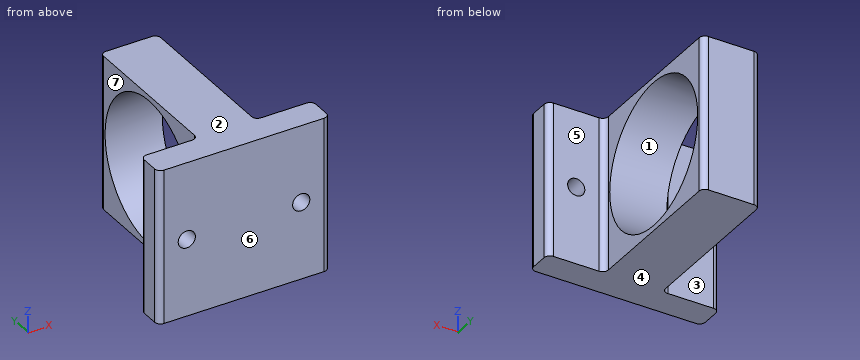
from build123d import *

# Parameters (mm, degrees)
BOSS_EXTRUDE1_DEPTH = 27
CUT_EXTRUDE1_REACH  = 45.738
SKETCH2_R           = 12.6
CUT_EXTRUDE2_REACH  = 47.2
SKETCH3_R           = 1.5


with BuildPart() as part:
    # Sketch1 → Boss-Extrude1 (new body)
    with BuildSketch(Plane.XY):
        with BuildLine():
            Line((-14, 0), (-6, 0))
            ThreePointArc((-6, 0), (-5.292893219, 0.292893219), (-5, 1))
            Line((-5, 1), (-5, 27))
            ThreePointArc((-5, 27), (-4.707106781, 27.707106781), (-4, 28))
            Line((-4, 28), (4, 28))
            ThreePointArc((4, 28), (4.707106781, 27.707106781), (5, 27))
            Line((5, 27), (5, 1))
            ThreePointArc((5, 1), (5.292893219, 0.292893219), (6, 0))
            Line((6, 0), (14, 0))
            ThreePointArc((14, 0), (14.707106781, -0.292893219), (15, -1))
            Line((15, -1), (15, -4))
            ThreePointArc((15, -4), (14.707106781, -4.707106781), (14, -5))
            Line((14, -5), (-14, -5))
            ThreePointArc((-14, -5), (-14.707106781, -4.707106781), (-15, -4))
            Line((-15, -4), (-15, -1))
            ThreePointArc((-15, -1), (-14.707106781, -0.292893219), (-14, 0))
        make_face()
    extrude(amount=BOSS_EXTRUDE1_DEPTH)

    # Sketch2 → Cut-Extrude1 (cut, up to next)
    with BuildSketch(Plane(origin=(5, 0, 0), x_dir=(0, 0, -1), z_dir=(1, 0, 0)), mode=Mode.PRIVATE) as cut_extrude1_sk1:
        with Locations(Location((-13.5, 14, 0), (0, 0, 90))):
            Circle(SKETCH2_R)
    cut_extrude1_tool1 = extrude(cut_extrude1_sk1.sketch, amount=-CUT_EXTRUDE1_REACH, mode=Mode.PRIVATE) & part.part
    add(cut_extrude1_tool1.solids().sort_by_distance((5, 14, 13.5))[0], mode=Mode.SUBTRACT)

    # Sketch3 → Cut-Extrude2 (cut, up to next)
    with BuildSketch(Plane.XZ.offset(5), mode=Mode.PRIVATE) as cut_extrude2_sk1:
        with Locations((-10, 13.5)):
            Circle(SKETCH3_R)
    cut_extrude2_tool1 = extrude(cut_extrude2_sk1.sketch, amount=-CUT_EXTRUDE2_REACH, mode=Mode.PRIVATE) & part.part
    # Sketch3 → Cut-Extrude2 (cut, up to next)
    with BuildSketch(Plane.XZ.offset(5), mode=Mode.PRIVATE) as cut_extrude2_sk2:
        with Locations(Location((10, 13.5, 0), (0, 0, 270))):
            Circle(SKETCH3_R)
    cut_extrude2_tool2 = extrude(cut_extrude2_sk2.sketch, amount=-CUT_EXTRUDE2_REACH, mode=Mode.PRIVATE) & part.part
    add(cut_extrude2_tool1.solids().sort_by_distance((-10, -5, 13.5))[0], mode=Mode.SUBTRACT)
    add(cut_extrude2_tool2.solids().sort_by_distance((10, -5, 13.5))[0], mode=Mode.SUBTRACT)


solid = part.part
Geometry check sheet. Reference: the model listing, model coordinates, mm. Face numbers are marked on the shaded views. A direction names the side the tool comes from. Coordinates: 2 decimals unless noted, no trailing zeros. Write each loop counter-clockwise with the first axis right and the second up, starting at its lowest first coordinate (ties: lowest second). Pieces come first, ordered by that corner, then holes. Notation, with made-up numbers: (-22, -18) -> (3, -18) arc R15 ccw to (3, -4) -> close; hole circle Ø3 at (31.25, -0.5). An arc over 180 degrees is marked (long way). One line per question, with ' | ' between items.
1. Cross-section at A-A on x = -10. Record the cut outline in (y, z).
Answers:
outline: (-5, 0) -> (0, 0) -> (0, 12) -> (-5, 12) -> close; (-5, 15) -> (0, 15) -> (0, 27) -> (-5, 27) -> close
2. Set-up check for the marked faces 5, 6 and 7: record each of +Z, -Z, +X, -X, +Y, -Y from which the full face is reachable in a straight line by a thin tool's end or side.
Answers:
face 5: +Z, -Z, +X, +Y | face 6: +Z, -Z, +X, -X, -Y | face 7: +Z, -Z, -X, +Y
3. Cross-section at D-D on z = 4.5. Record the cut outline in (x, y).
Answers:
outline: (-15, -4) arc R1 ccw to (-14, -5) -> (14, -5) arc R1 ccw to (15, -4) -> (15, -1) arc R1 ccw to (14, 0) -> (6, 0) arc R1 cw to (5, 1) -> (5, 5.18) -> (-5, 5.18) -> (-5, 1) arc R1 cw to (-6, 0) -> (-14, 0) arc R1 ccw to (-15, -1) -> close; (-5, 22.82) -> (5, 22.82) -> (5, 27) arc R1 ccw to (4, 28) -> (-4, 28) arc R1 ccw to (-5, 27) -> close
4. Depth check by flat-ended pin: pin 1 Ø9 at (x, z) = (-10, 19) entering from +Y; pin 2 Ø1.5 at (x, y) = (-3, 0.5) entering from -Z; pin 3 Ø6.5 at (x, z) = (8, 18) entering from +Y. Enter the tip coordinate at first touch or a pass-through.
Answers:
pin 1: stops at y = 0.13 | pin 2: stops at z = 0 | pin 3: stops at y = 27.66
5. Cross-section at C-C on y = 18. Record the cut outline in (x, z).
Answers:
outline: (-5, 0) -> (5, 0) -> (5, 1.55) -> (-5, 1.55) -> close; (-5, 25.45) -> (5, 25.45) -> (5, 27) -> (-5, 27) -> close
6. Cross-section at B-B on z = 13.5. Record the cut outline in (x, y).
Answers:
outline: (-15, -4) arc R1 ccw to (-14, -5) -> (-11.5, -5) -> (-11.5, 0) -> (-14, 0) arc R1 ccw to (-15, -1) -> close; (-8.5, -5) -> (8.5, -5) -> (8.5, 0) -> (6, 0) arc R1 cw to (5, 1) -> (5, 1.4) -> (-5, 1.4) -> (-5, 1) arc R1 cw to (-6, 0) -> (-8.5, 0) -> close; (-5, 26.6) -> (5, 26.6) -> (5, 27) arc R1 ccw to (4, 28) -> (-4, 28) arc R1 ccw to (-5, 27) -> close; (11.5, -5) -> (14, -5) arc R1 ccw to (15, -4) -> (15, -1) arc R1 ccw to (14, 0) -> (11.5, 0) -> close
7. Draft check along Z on the marked faces 1, 2, 3 and 4. Enter one of: +Z half, -Z half, draft (parallel to the pull), parting line (faces both ways), or undercut.
Answers:
face 1: undercut | face 2: +Z half | face 3: draft | face 4: -Z half
8. Thickness scan on probe 1 along Z at (x, y) = (1, 14); probe 2 along Z at (x, y) = (-10, -3.4); probe 3 along Y at (x, z) = (-2.25, 20.5). Record the ranges inside material, lowest first. Write a range as from..to.
Answers:
probe 1: z = 0..0.9, 26.1..27 | probe 2: z = 0..12, 15..27 | probe 3: y = -5..3.52, 24.48..28
